Here's the drawing with two shaded views (mm, measured from the low corner). I have some questions. Round coordinates to 2 decimals unless told otherwise and drop trailing zeros. Loops run counter-clockwise (first coordinate to the right, second up) from the corner with the lowest first, then second, coordinate; pieces in that order, holes last.
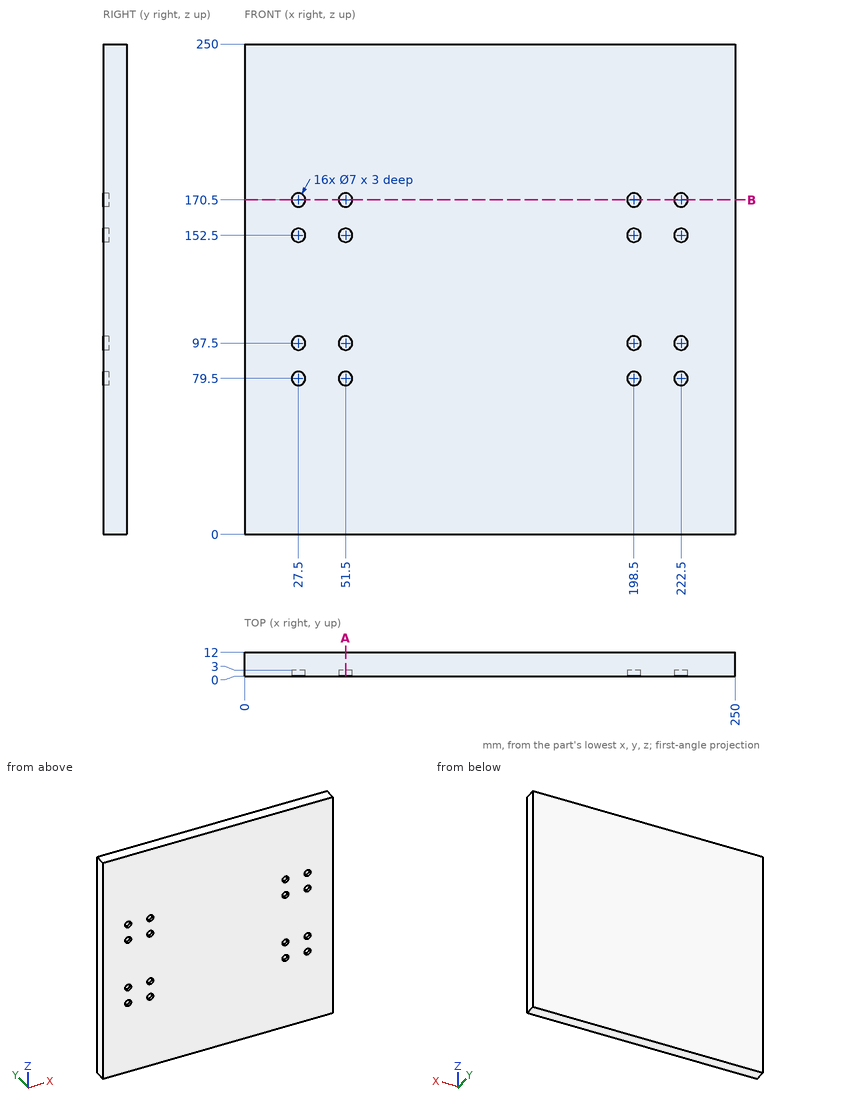
Item 1: If we section it at A-A, the plane x = 51.5: Please give me the cut outline in (y, z).
Results list:
outline: (0, 0) - (12, 0) - (12, 250) - (0, 250) - (0, 174) - (3, 174) - (3, 167) - (0, 167) - (0, 156) - (3, 156) - (3, 149) - (0, 149) - (0, 101) - (3, 101) - (3, 94) - (0, 94) - (0, 83) - (3, 83) - (3, 76) - (0, 76) - close
Item 2: Will this pin go through, and if not, where does the flat tip stop? pin 1 (5.5 mm diameter, centred on x = 198.5, z = 79.5, fed in from -Y).
Results list:
pin 1: stops at y = 3
Item 3: If we section it at B-B, the plane z = 170.5: Please give me the cut outline in (x, y).
Results list:
outline: (0, 0) - (24, 0) - (24, 3) - (31, 3) - (31, 0) - (48, 0) - (48, 3) - (55, 3) - (55, 0) - (195, 0) - (195, 3) - (202, 3) - (202, 0) - (219, 0) - (219, 3) - (226, 3) - (226, 0) - (250, 0) - (250, 12) - (0, 12) - close
Item 4: If I drill on line 1 along Z through (x, y) = (222.5, 1.2); line 2 along X through (y, z) = (1.6, 152.5); line 3 along Y through (x, z) = (27, 80), over which ranges is the centre line in solid material (lowest first)?
Results list:
line 1: z = 0 to 76, 83 to 94, 101 to 149, 156 to 167, 174 to 250
line 2: x = 0 to 24, 31 to 48, 55 to 195, 202 to 219, 226 to 250
line 3: y = 3 to 12
